Build history of the part. All positions in model axes, mm. A direction names the side the tool comes from. Give positions to 0.01 mm unless a question says otherwise; leave off trailing zeros. Order: outer loops, then holes, each group sorted by start corner. A loop starts at its lowest first (then second) coordinate and runs counter-clockwise, first axis right, second up. Notation, with made-up numbers: (69.5, 36) -> (123.5, 36) arc R29 cw to (123.5, 59) -> close; hole circle Ø8 at (0.25, -14.75). An arc over 180 degrees is marked (long way). One line per item, written item: value. Start each with the question number.
(1) Saw through at D-D on x = 37. Give the cut face in (y, z), plus the area to 3 significant figures.
(2) Saw through at C-C on z = -36.5. Give the cut face in (x, y), plus the area to 3 significant figures.
(3) Two-plate mould, pull along X, no slides. Class faces 1 (the flat face through (30, 25, -20)), 2 (the flat face through (76, 15, -30)), 3 (the cylindrical face through (42, 29, -20)), 4 (the flat face through (70, 25, -20)): +X half, -X half, draft (parallel to the pull), parting line (faces both ways), or undercut.
(4) Pin check, flat tips, straight feed: pin 1 (5 mm diameter, centred on x = 103, z = -34.5, fed in from +Y); pin 2 (10 mm diameter, centred on y = 24.5, z = -14, fed in from +X); pin 3 (1.5 mm diameter, centred on x = 33.5, z = -44.5, fed in from -Y); pin 4 (10 mm diameter, centred on y = 20.5, z = -27, fed in from -X). Stop position of each tip, or through.
(5) Saw through at B-B on x = 50. Give the cut face in (y, z), plus the area to 3 significant figures.
(6) Probe line 1 (Y direction, x = 50, z = -17); line 2 (X direction, y = 34.5, z = -21); line 3 (Z direction, x = 66.5, y = 31). List the from-to ranges inside material, lowest first.
(7) Which spindle directions (+Z, -Z, +X, -X, +Y, -Y) get a long thin tool onto all of the face, cutting with end or side? Do faces 5 (the flat face through (62, 16, 0)), 6 (the flat face through (50, 22, -40)). Say none if no direction does.
(8) Saw through at A-A on y = 27. Give the cut face in (x, z), plus the area to 3 significant figures.
```python
from build123d import *

# Parameters (mm, degrees)
SKETCH1_W           = 125
SKETCH1_H           = 15
BOSS_EXTRUDE1_DEPTH = 60
SKETCH1_3_R         = 10
BOSS_EXTRUDE2_DEPTH = 40


with BuildPart() as part:
    # Sketch1 → Boss-Extrude1 (new body)
    with BuildSketch(Plane.XY):
        with Locations((62.5, 7.5)):
            Rectangle(SKETCH1_W, SKETCH1_H)
    extrude(amount=-BOSS_EXTRUDE1_DEPTH)

    # Sketch1_3 → Boss-Extrude2 (add)
    with BuildSketch(Plane.XY):
        with BuildLine():
            Line((30, 35), (30, 15))
            Line((30, 15), (70, 15))
            Line((70, 15), (70, 35))
            ThreePointArc((70, 35), (50, 55), (30, 35))
        make_face()
        with Locations((50, 35)):
            Circle(SKETCH1_3_R, mode=Mode.SUBTRACT)
    extrude(amount=-BOSS_EXTRUDE2_DEPTH)


solid = part.part
```
Results below:
1. outline: (0, -60) -> (15, -60) -> (15, -40) -> (50.2, -40) -> (50.2, 0) -> (0, 0) -> close
1. area: 2,310 mm²
2. outline: (0, 0) -> (125, 0) -> (125, 15) -> (70, 15) -> (70, 35) arc R20 ccw to (30, 35) -> (30, 15) -> (0, 15) -> close; hole circle Ø20 at (50, 35)
2. area: 2,990 mm²
3. face 1: -X half
3. face 2: draft
3. face 3: undercut
3. face 4: +X half
4. pin 1: stops at y = 15
4. pin 2: stops at x = 70
4. pin 3: stops at y = 0
4. pin 4: stops at x = 30
5. outline: (0, -60) -> (15, -60) -> (15, -40) -> (25, -40) -> (25, 0) -> (0, 0) -> close; (45, -40) -> (55, -40) -> (55, 0) -> (45, 0) -> close
5. area: 1,700 mm²
6. line 1: y = 0 to 25, 45 to 55
6. line 2: x = 30 to 40.01, 59.99 to 70
6. line 3: z = -40 to 0
7. face 5: +Z, +X, -X, +Y, -Y
7. face 6: -Z, +X, -X, +Y
8. outline: (30, -40) -> (44, -40) -> (44, 0) -> (30, 0) -> close; (56, -40) -> (70, -40) -> (70, 0) -> (56, 0) -> close
8. area: 1,120 mm²
